Autodesk Inventor part; units mm, degrees
ref_plane "YZ Plane" through (0, 0, 0) normal (1, 0, 0) x (0, 1, 0)
ref_plane "XZ Plane" through (0, 0, 0) normal (0, 1, 0) x (-1, 0, 0)
ref_plane "XY Plane" through (0, 0, 0) normal (0, 0, 1) x (1, 0, 0)
sketch "Sketch1" plane through (0, 0, 0) normal (0, 1, 0) x (-1, 0, 0)
  line L0 (-25, 25) -> (25, 25)
  line L1 (25, 25) -> (25, -25)
  line L2 (25, -25) -> (-25, -25)
  line L3 (-25, -25) -> (-25, 25)
  line L4 (-25, 25) -> (25, -25) construction
  line L5 (25, 25) -> (-25, -25) construction
  line L6 (-17.4, 17.4) -> (17.4, 17.4)
  line L7 (17.4, 17.4) -> (17.4, -17.4)
  line L8 (17.4, -17.4) -> (-17.4, -17.4)
  line L9 (-17.4, -17.4) -> (-17.4, 17.4)
  line L10 (-17.4, 17.4) -> (17.4, -17.4) construction
  line L11 (17.4, 17.4) -> (-17.4, -17.4) construction
  point P0 (0, 0)
  dimension "d0" = 50
  dimension "d1" = 50
  dimension "d2" = 34.8
  dimension "d3" = 34.8
extrude "Extrusion1" add sketch "Sketch1" along normal blind 5
extrude "Extrusion2" add sketch "Sketch1" along normal blind 15 contours L6 L7 L8 L9
sketch "Sketch3" plane through (0, 15, 0) normal (0, 1, 0) x (1, 0, 0)
  point P0 (0, 0)
ref_plane "Work Plane6" through (0, 5, 17.4) normal (-1, 0, 0) x (0, 0, 1)
ref_plane "Work Plane7" through (-17.4, 5, 0) normal (0, 0, 1) x (1, 0, 0)
sketch "Sketch6" plane through (0, 0, 0) normal (0, -1, 0) x (1, 0, 0)
  line L0 (-25, 25) -> (25, 25)
  line L1 (-5, -25) -> (5, -25)
  line L2 (5, -25) -> (5, 25)
  line L3 (5, 25) -> (-5, 25)
  line L4 (-5, 25) -> (-5, -25)
  line L5 (-5, -25) -> (5, 25) construction
  line L6 (5, -25) -> (-5, 25) construction
  line L7 (25, 25) -> (25, -25)
  line L8 (-25, -5) -> (25, -5)
  line L9 (25, -5) -> (25, 5)
  line L10 (25, 5) -> (-25, 5)
  line L11 (-25, 5) -> (-25, -5)
  line L12 (-25, -5) -> (25, 5) construction
  line L13 (25, -5) -> (-25, 5) construction
  point P0 (0, 0)
  point P1 (-5, -5)
  point P2 (5, -5)
  point P3 (5, 5)
  point P4 (-5, 5)
  dimension "d14" = 10
extrude "Extrusion5" add sketch "Sketch6" along normal blind 2 contours L0 L2 L10 L4 | L10 L2 L8 L4 | L4 L8 L11 L10 | L10 L7 L8 L2 | L8 L2 L1 L4
sketch "Sketch7" plane through (-25, 0, 25) normal (-1, 0, 0) x (0, 0, 1)
  line L0 (-20, -2) -> (-30, -2)
  line L1 (-7.6, 5) -> (-42.4, 5)
  line L2 (-20, -2) -> (-30, -2)
  line L3 (-30, -2) -> (-30, 5)
  line L4 (-30, 5) -> (-20, 5)
  line L5 (-20, 5) -> (-20, -2)
  point P0 (-25, 0)
  dimension "d17" = 10
extrude "Extrusion6" add sketch "Sketch7" along normal blind 2
mirror "Mirror4" about plane through (0, 5, 17.4) normal (-1, 0, 0) of "Extrusion6"
sketch "Sketch8" plane through (25, 5, -25) normal (0, 0, -1) x (-1, 0, 0)
  line L0 (30, -7) -> (20, -7)
  line L1 (0, 0) -> (50, 0)
  line L2 (20, -7) -> (30, -7)
  line L3 (30, -7) -> (30, 0)
  line L4 (30, 0) -> (20, 0)
  line L5 (20, 0) -> (20, -7)
  point P0 (25, -5)
  dimension "d20" = 10
extrude "Extrusion7" add sketch "Sketch8" along normal blind 2
mirror "Mirror5" about plane through (-17.4, 5, 0) normal (0, 0, 1) of "Extrusion7"
sketch "Sketch9" plane through (0, 0, 0) normal (0, -1, 0) x (1, 0, 0)
  line L0 (-27, 27) -> (27, 27)
  line L1 (27, 27) -> (27, -27)
  line L2 (27, -27) -> (-27, -27)
  line L3 (-27, -27) -> (-27, 27)
  line L4 (-27, 27) -> (27, -27) construction
  line L5 (27, 27) -> (-27, -27) construction
  point P0 (0, 0)
  dimension "d24" = 54
  dimension "d25" = 54
extrude "Extrusion8" cut sketch "Sketch9" along normal blind 6.75
sketch "Sketch10" plane through (0, 15, 0) normal (0, 1, 0) x (1, 0, 0)
  line L0 (12.5, -12.5) -> (-12.5, -12.5)
  line L1 (-12.5, -12.5) -> (-12.5, 12.5)
  line L2 (-12.5, 12.5) -> (12.5, 12.5)
  line L3 (12.5, 12.5) -> (12.5, -12.5)
  line L4 (12.5, -12.5) -> (-12.5, 12.5) construction
  line L5 (-12.5, -12.5) -> (12.5, 12.5) construction
  point P0 (0, 0)
  dimension "d28" = 25
  dimension "d29" = 25
extrude "Extrusion9" cut sketch "Sketch10" against normal blind 11.45
sketch "Sketch11" plane through (-17.4, 5, 17.4) normal (-1, 0, 0) x (0, 0, 1)
  line L0 (-17.5, 0.0162) -> (-17.5, 3.0162)
  circle A0 centre (-17.5, 3.0162) radius 1.75
  point P0 (-17.4, -5)
  dimension "d33" = 3
  dimension "d34" = 3.5
extrude "Extrusion10" cut sketch "Sketch11" against normal through all
sketch "Sketch12" plane through (17.4, 5, -17.4) normal (0, 0, -1) x (-1, 0, 0)
  line L0 (17.5, -0.0575) -> (17.5, 2.9425)
  circle A0 centre (17.5, 2.9425) radius 1.75
  point P0 (17.4, -5)
  dimension "d37" = 3
  dimension "d38" = 3.5
extrude "Extrusion11" cut sketch "Sketch12" against normal blind 3.5
mirror "Mirror6" about plane through (-17.4, 5, 0) normal (0, 0, 1) of "Extrusion11"
sketch "Sketch13" plane through (0, 15, 0) normal (0, 1, 0) x (1, 0, 0)
  line L0 (5, -25) -> (25, -25)
  line L1 (-25, 25) -> (25, 25)
  line L2 (25, 25) -> (25, -25)
  line L3 (25, -25) -> (-25, -25)
  line L4 (-25, -25) -> (-25, 25)
  line L5 (-25, 25) -> (25, -25) construction
  line L6 (25, 25) -> (-25, -25) construction
  point P0 (0, 0)
  point P1 (5, -25)
extrude "Extrusion12" cut sketch "Sketch13" against normal blind 3
sketch "Sketch14" plane through (27, 0, -5) normal (1, 0, 0) x (0, 0, -1)
  line L0 (12.4, 5) -> (-22.4, 5)
  line L1 (-15, 0) -> (5, 0)
  line L2 (5, 0) -> (5, 5)
  line L3 (5, 5) -> (-15, 5)
  line L4 (-15, 5) -> (-15, 0)
  line L5 (-15, 0) -> (5, 5) construction
  line L6 (5, 0) -> (-15, 5) construction
  point P0 (-5, 0)
  point P1 (-5, 2.5)
  dimension "d43" = 20
extrude "Extrusion13" cut sketch "Sketch14" against normal blind 4
pattern_circular "Circular Pattern1" count 4 over 360 about axis through (0, -10, 0) along (0, 1, 0) of "Extrusion13"
properties part number "Pokrywka"
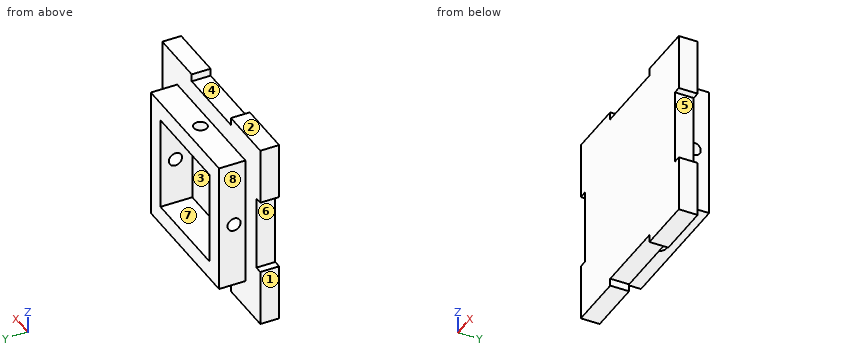
Check sheet for the modelled part. Datum: model origin and axes. Units: mm. Face numbers are marked on the shaded views. A direction names the side the tool comes from. Give positions to 0.01 mm unless a question says otherwise; leave off trailing zeros. Write each loop counter-clockwise with the first axis right and the second up, starting at its lowest first coordinate (ties: lowest second). Pieces come first, ordered by that corner, then holes.
Item 1: Scan lines: L1, parallel to Y at x = 15.7, z = -0.1; L2, parallel to Z at x = -10, y = 7. Record each from-to range of solid material in increasing order.
Item 2: Cross-section at A-A (z = -0.1). Enter the section's corners in (x, y).
Item 3: Draft check along Z on the marked faces 1, 2 and 3. Enter one of: released by +Z, released by -Z, zero draft, split by the parting line, or undercut.
Item 4: Cross-section at C-C (y = 4.25). Enter the section's corners in (x, z), and give its area (4 significant figures).
Item 5: Cross-section at D-D (z = -7). Enter the section's corners in (x, y), and give its area (3 significant figures).
Item 6: Access from +Z, -Z, +X, -X, +Y, -Y to the whole of each face (thin tool, end or side, straight path). Record for the marked faces 4, 5, 6, 7 and 8.
Item 7: Cross-section at B-B (x = -0.1). Enter the section's corners in (y, z), and give its area (3 significant figures).
Item 8: Gauge pin test, flat ends, axial feed: pin 1 (5.5 mm diameter, centred on x = -2.5, y = 3.5, fed in from +Z); pin 2 (1.5 mm diameter, centred on x = -2.5, y = 3.5, fed in from -Z); pin 3 (4.5 mm diameter, centred on y = 8.02, z = -0.1, fed in from +X); pin 4 (6 mm diameter, centred on x = -19.5, z = -5.5, fed in from +Y). Record the tip position at first contact, or that the pin passes through.
Report:
1. L1: y = 0 to 6.27, 9.77 to 12
1. L2: z = -17.4 to -12.5, 12.5 to 17.4
2. outline: (-23, 0) - (23, 0) - (23, 5) - (17.4, 5) - (17.4, 6.27) - (12.5, 6.27) - (12.5, 3.55) - (-12.5, 3.55) - (-12.5, 6.27) - (-17.4, 6.27) - (-17.4, 5) - (-23, 5) - close; (-17.4, 9.77) - (-12.5, 9.77) - (-12.5, 12) - (-17.4, 12) - close; (12.5, 9.77) - (17.4, 9.77) - (17.4, 12) - (12.5, 12) - close
3. face 1: zero draft
3. face 2: released by +Z
3. face 3: undercut
4. outline: (-25, -25) - (-10, -25) - (-10, -23) - (10, -23) - (10, -25) - (25, -25) - (25, -10) - (23, -10) - (23, 10) - (25, 10) - (25, 25) - (10, 25) - (10, 23) - (-10, 23) - (-10, 25) - (-25, 25) - (-25, 10) - (-23, 10) - (-23, -10) - (-25, -10) - close; hole (-12.5, -12.5) - (12.5, -12.5) - (12.5, 12.5) - (-12.5, 12.5) - close
4. area: 1,715 mm2
5. outline: (-23, 0) - (23, 0) - (23, 5) - (17.4, 5) - (17.4, 12) - (12.5, 12) - (12.5, 3.55) - (-12.5, 3.55) - (-12.5, 12) - (-17.4, 12) - (-17.4, 5) - (-23, 5) - close
5. area: 262 mm2
6. face 4: +Z, +Y, -Y
6. face 5: +X, +Y, -Y
6. face 6: -X, +Y, -Y
6. face 7: +Y
6. face 8: +Z, -Z, -X, +Y
7. outline: (0, -23) - (5, -23) - (5, -17.4) - (6.19, -17.4) - (6.19, -13.9) - (9.69, -13.9) - (9.69, -17.4) - (12, -17.4) - (12, -12.5) - (3.55, -12.5) - (3.55, 12.5) - (12, 12.5) - (12, 17.4) - (9.69, 17.4) - (9.69, 13.9) - (6.19, 13.9) - (6.19, 17.4) - (5, 17.4) - (5, 23) - (0, 23) - close
7. area: 238 mm2
8. pin 1: stops at z = 23
8. pin 2: stops at z = -23
8. pin 3: stops at x = 17.4
8. pin 4: stops at y = 12
